Input: part model. Units: mm. Frame: model coordinates. A direction names the side the tool comes from. Coordinates: 2 decimals unless noted, no trailing zeros. Write each loop counter-clockwise with the first axis right and the second up, starting at its lowest first coordinate (ties: lowest second). Pieces come first, ordered by that corner, then holes. Notation, with made-up numbers: (31.5, -36.75) - (37.5, -36.75) arc R14 cw to (37.5, -24.75) - close; hole circle Ø1 at (29, 80.5). An arc over 180 degrees is marked (long way). One line per question, with ' | ' between items. Start each with the question number.
1) Reachability of faces 1 (the flat face through (-5, -700, -85)), 2 (the flat face through (-5, -74, 85)), 3 (the flat face through (5, -74, -85)), 4 (the flat face through (85, -74, 5)), 5 (the flat face through (0, -125, 90)) from +Z, -Z, +X, -X, +Y, -Y: full face, straight path, thin tool, end or side. Return the list, or none.
2) Line query: line 1 (Z direction, x = -75, y = 4); line 2 (Z direction, x = 75, y = -741.75); line 3 (Y direction, x = -23, z = 50). Output: solid intervals per line, ascending.
3) First-contact query: P1, Ø3, axis at y = -535, z = 64, coming from the -X side; P2, Ø1, axis at y = -345.5, z = -47, coming from the -X side; P3, Ø15, axis at y = -43, z = 86.5, coming from the -X side. Flat tips, straight axial feed; report the tip coordinate or a pass-through.
4) Section query A-A on z = -45. Return loops of the section in (x, y), and give its area (3 significant figures).
5) Section query B-B on x = 20.5. Return loops of the section in (y, z).
6) Draft query along Z for faces 6 (the cylindrical face through (-86, 5, -75)), 7 (the flat face through (-5, -74, -85)), 8 (the flat face through (0, -681, 90)). Return one class per face: released by +Z, released by -Z, zero draft, split by the parting line, or undercut.
7) Section query C-C on y = -535.5. Return loops of the section in (x, z).
```python
from build123d import *

# Parameters (mm, degrees)
F0_R          = 70
F0_R_2        = 65
F1_DEPTH      = 736
F2_W          = 200
F2_H          = 200
F2_R          = 11
F3_DEPTH      = 10
F4_W          = 30.1787997812
F4_H          = 10
F4_W_2        = 10
F4_H_2        = 30.1787997812
F5_DEPTH      = 150
F6_T1_DEPTH   = 269.311363913
F6_T3_DEPTH   = 269.311363913
F6_T8_DEPTH   = 269.311363913
F6_S9_R       = 70
F6_T10_DEPTH  = 139
F8_W          = 200
F8_H          = 200
F8_R          = 8.5
F9_DEPTH      = 10
F10_W         = 10
F10_H         = 30.1787997812
F10_W_2       = 30.1787997812
F10_H_2       = 10
F11_DEPTH     = 80
F12_T1_DEPTH  = 269.311363913
F12_T3_DEPTH  = 269.311363913
F12_T8_DEPTH  = 269.311363913
F12_S9_R      = 70
F12_T10_DEPTH = 139
F12_T14_DEPTH = 269.311363913
F12_S15_R     = 70
F12_T16_DEPTH = 139


# Not quite as in the source:
# - a fillet or chamfer that OpenCascade refuses, or shapes differently, is made with other operations: its cross-section is extruded or revolved along the edge and cut away or added


with BuildPart() as f1:
    # F0 (on Front) → F1 (new body)
    with BuildSketch(Plane.XZ):
        Circle(F0_R)
        Circle(F0_R_2, mode=Mode.SUBTRACT)
    extrude(amount=F1_DEPTH)

    # F2 (on Front) → F3 (join)
    with BuildSketch(Plane.XZ):
        Rectangle(F2_W, F2_H)
        with Locations((-75, -75)):
            Circle(F2_R, mode=Mode.SUBTRACT)
        with Locations((75, -75)):
            Circle(F2_R, mode=Mode.SUBTRACT)
        with Locations((-75, 75)):
            Circle(F2_R, mode=Mode.SUBTRACT)
        with Locations((75, 75)):
            Circle(F2_R, mode=Mode.SUBTRACT)
    extrude(amount=-F3_DEPTH)

    # F4 (on Front) → F5 (join)
    with BuildSketch(Plane.XZ):
        with Locations((-84.9106001094, 0)):
            Rectangle(F4_W, F4_H)
        with Locations((0, 84.9106001094)):
            Rectangle(F4_W_2, F4_H_2)
        with Locations((84.9106001094, 0)):
            Rectangle(F4_W, F4_H)
        with Locations((0, -84.9106001094)):
            Rectangle(F4_W_2, F4_H_2)
    extrude(amount=F5_DEPTH)

    # F6: chamfer of 50 x 20 on 4 edges, made by hand

    # F6_s2 → F6_t1 (cut)
    with BuildSketch(Plane.YZ.offset(-134.6556819565)):
        Polygon((-100, 100), (-150, 80), (-150, 100), align=None)
        Polygon((-100, -100), (-150, -80), (-150, -100), align=None)
    extrude(amount=F6_T1_DEPTH, mode=Mode.SUBTRACT)

    # F6_s4 → F6_t3 (cut)
    with BuildSketch(Plane.XY.offset(-134.6556819565)):
        Polygon((100, -100), (80, -150), (100, -150), align=None)
    extrude(amount=F6_T3_DEPTH, mode=Mode.SUBTRACT)


with BuildPart() as f6_tool6:
    # F6_s7 → F6_t8 (new body)
    with BuildSketch(Plane.XY.offset(134.6556819565)):
        Polygon((-100, -130), (-50, -150), (-100, -150), align=None)
    extrude(amount=-F6_T8_DEPTH)

    # F6_s9 → F6_t10 (cut, symmetric)
    with BuildSketch(Plane.XZ.offset(140)):
        Circle(F6_S9_R)
    extrude(amount=F6_T10_DEPTH, both=True, mode=Mode.SUBTRACT)


with BuildPart() as f1_1:
    add(f1.part)

    # F6_t5: cut F6_tool6
    add(f6_tool6.part, mode=Mode.SUBTRACT)

    # F8 (on offset) → F9 (join)
    with BuildSketch(Plane.XZ.offset(736)):
        Rectangle(F8_W, F8_H)
        with Locations((-75, -75)):
            Circle(F8_R, mode=Mode.SUBTRACT)
        with Locations((75, -75)):
            Circle(F8_R, mode=Mode.SUBTRACT)
        with Locations((-75, 75)):
            Circle(F8_R, mode=Mode.SUBTRACT)
        with Locations((75, 75)):
            Circle(F8_R, mode=Mode.SUBTRACT)
    extrude(amount=F9_DEPTH)

    # F10 (on face) → F11 (join)
    with BuildSketch(Plane(origin=(0, -736, 0), x_dir=(-1, 0, 0), z_dir=(0, 1, 0))):
        with Locations((0, 84.9106001094)):
            Rectangle(F10_W, F10_H)
        with Locations((84.9106001094, 0)):
            Rectangle(F10_W_2, F10_H_2)
        with Locations((0, -84.9106001094)):
            Rectangle(F10_W, F10_H)
        with Locations((-84.9106001094, 0)):
            Rectangle(F10_W_2, F10_H_2)
    extrude(amount=F11_DEPTH)

    # F12: chamfer of 20 x 50 on 4 edges, made by hand

    # F12_s2 → F12_t1 (cut)
    with BuildSketch(Plane.YZ.offset(-134.6556819565)):
        Polygon((-706, 100), (-656, 80), (-656, 100), align=None)
    extrude(amount=F12_T1_DEPTH, mode=Mode.SUBTRACT)

    # F12_s4 → F12_t3 (cut)
    with BuildSketch(Plane.XY.offset(-134.6556819565)):
        Polygon((100, -706), (80, -656), (100, -656), align=None)
    extrude(amount=F12_T3_DEPTH, mode=Mode.SUBTRACT)


with BuildPart() as f12_tool6:
    # F12_s7 → F12_t8 (new body)
    with BuildSketch(Plane.XY.offset(-134.6556819565)):
        Polygon((-100, -676), (-50, -656), (-100, -656), align=None)
    extrude(amount=F12_T8_DEPTH)

    # F12_s9 → F12_t10 (cut, symmetric)
    with BuildSketch(Plane.XZ.offset(666)):
        Circle(F12_S9_R)
    extrude(amount=F12_T10_DEPTH, both=True, mode=Mode.SUBTRACT)


with BuildPart() as f1_2:
    add(f1_1.part)

    # F12_t5: cut F12_tool6
    add(f12_tool6.part, mode=Mode.SUBTRACT)


with BuildPart() as f12_tool12:
    # F12_s13 → F12_t14 (new body)
    with BuildSketch(Plane.YZ.offset(134.6556819565)):
        Polygon((-676, -100), (-656, -50), (-656, -100), align=None)
    extrude(amount=-F12_T14_DEPTH)

    # F12_s15 → F12_t16 (cut, symmetric)
    with BuildSketch(Plane.XZ.offset(666)):
        Circle(F12_S15_R)
    extrude(amount=F12_T16_DEPTH, both=True, mode=Mode.SUBTRACT)


with BuildPart() as f1_3:
    add(f1_2.part)

    # F12_t11: cut F12_tool12
    add(f12_tool12.part, mode=Mode.SUBTRACT)


solid = f1_3.part
```
Answer key:
1) face 1: -Z, -X | face 2: +Z, -X | face 3: -Z, +X | face 4: +Z, +X | face 5: +Z, +X, -X
2) line 1: -100 to -86, -64 to 64, 86 to 100 | line 2: -100 to -83.5, -66.5 to 66.5, 83.5 to 100 | line 3: -746 to -736, 0 to 10
3) P1: x = -31.52 | P2: x = -52.32 | P3: x = -5
4) outline: (-100, -746) - (100, -746) - (100, -736) - (53.62, -736) - (53.62, 0) - (100, 0) - (100, 10) - (-100, 10) - (-100, 0) - (-53.62, 0) - (-53.62, -736) - (-100, -736) - close; hole (-46.9, -736) - (46.9, -736) - (46.9, 0) - (-46.9, 0) - close | area: 13,900 mm²
5) outline: (-746, -100) - (-736, -100) - (-736, -66.93) - (0, -66.93) - (0, -100) - (10, -100) - (10, 100) - (0, 100) - (0, 66.93) - (-736, 66.93) - (-736, 100) - (-746, 100) - close; hole (-736, -61.68) - (0, -61.68) - (0, 61.68) - (-736, 61.68) - close
6) face 6: undercut | face 7: zero draft | face 8: released by +Z
7) outline: circle Ø140 at (0, 0); hole circle Ø130 at (0, 0)
